Autodesk Inventor part; units mm, degrees
ref_plane "YZ Plane" through (0, 0, 0) normal (1, 0, 0) x (0, 1, 0)
ref_plane "XZ Plane" through (0, 0, 0) normal (0, 1, 0) x (-1, 0, 0)
ref_plane "XY Plane" through (0, 0, 0) normal (0, 0, 1) x (1, 0, 0)
sketch "스케치1" plane through (0, 0, 0) normal (0, 0, 1) x (1, 0, 0)
  arc A0 (0, 12.5) -> (-12.5, 0) centre (0, 0) ccw
  line L0 (0, 220.6094) -> (0, -371.145)
  line L1 (-77.086, -220) -> (-110, -35)
  line L2 (-110, -35) -> (-110, 15)
  spline S0 degree 2 poles (-110, 15) (-61.239, 69.4656) (0, 70) knots 0 0 0 1 1 1
  line L3 (-29.7943, 69.74) -> (29.7943, 70.26) construction
  line L4 (-12.5, 0) -> (-12.5, -190)
  line L5 (-12.5, -190) -> (-29.9689, -220)
  line L6 (-29.9689, -220) -> (-77.086, -220)
  arc A1 (12.5, 0) -> (0, 12.5) centre (0, 0) ccw
  line L7 (77.086, -220) -> (110, -35)
  line L8 (110, -35) -> (110, 15)
  spline S1 degree 2 poles (110, 15) (61.239, 69.4656) (0, 70) knots 0 0 0 1 1 1
  line L9 (29.7943, 69.74) -> (-29.7943, 70.26) construction
  line L10 (12.5, 0) -> (12.5, -190)
  line L11 (12.5, -190) -> (29.9689, -220)
  line L12 (29.9689, -220) -> (77.086, -220)
  point P0 (1.2114, -68.8044)
  point P1 (23.5091, 68.2027)
  point P2 (-23.4485, 67.5354)
  point P3 (-1.2114, -68.8044)
  point P4 (-23.5091, 68.2027)
  point P5 (23.4485, 67.5354)
  point P6 (0, 70)
  dimension "d0" = 25
  dimension "d3" = 110
  dimension "d4" = 50
  dimension "d5" = 190
  dimension "d8" = 70
  dimension "d25" = 290
extrude "Wheel Body Initial Extrusion" add sketch "스케치1" along normal mid plane 60
sketch "스케치4" plane through (-12.5, -190, 30) normal (1, 0, 0) x (0, 0, -1)
  line L0 (60, 190) -> (0, 190)
  line L1 (60, 190) -> (60, 0)
  line L2 (60, 0) -> (0, 0)
  line L3 (0, 0) -> (0, 190)
  line L4 (0, 190) -> (0, -93.6851)
  line L5 (23, 50) -> (10, 50)
  line L6 (10, 50) -> (10, -48.4584)
  line L7 (10, -10.6044) -> (23, -10.6044)
  line L8 (23, -10.6044) -> (23, -50.5115)
  line L9 (23, -50.5115) -> (0, -50.5115)
  line L10 (53, -93.6851) -> (53, 276.7845)
  line L11 (53, 190) -> (0, 190)
  line L12 (53, 259.8429) -> (0, 259.8429)
  line L13 (0, 259.8429) -> (0, 0)
  point P0 (30, 190)
  dimension "d18" = 13
  dimension "d19" = 140
  dimension "d20" = 7
sketch "스케치7" plane through (0, 0, 30) normal (0, 0, 1) x (1, 0, 0)
  line L0 (-103, -34.3822) -> (-71.2215, -213)
  line L1 (-71.2215, -213) -> (-34.8207, -213)
  line L2 (-29.9689, -220) -> (-77.086, -220)
  line L3 (-34.8207, -213) -> (-19.5, -189.0198)
  line L4 (-19.5, -189.0198) -> (-19.5, 0)
  line L5 (-103, -34.3822) -> (-103, 27.8234)
  line L6 (-103, 27.8234) -> (-55.0885, 51.7889) construction
  line L7 (-55.0885, 51.7889) -> (35.24, 53.8015) construction
  spline S0 degree 2 poles (-103, 27.8234) (-55.0885, 51.7889) (35.24, 53.8015) knots 1 1 1 2 2 2
  line L8 (12.5, -190) -> (12.5, 0)
  arc A0 (12.5, 0) -> (-12.5, 0) centre (0, 0) ccw
  line L9 (-110, 15) -> (-110, -35)
  line L10 (-110, -35) -> (-77.086, -220)
  line L11 (-12.5, -190) -> (-12.5, 0)
  arc A1 (0, 19.5) -> (-19.5, 0) centre (0, 0) ccw
  line L12 (138.0234, -13.4315) -> (72.0365, -213)
  line L13 (72.0365, -213) -> (34.8207, -213)
  line L14 (34.8207, -213) -> (19.5, -189.0198)
  line L15 (19.5, -189.0198) -> (19.5, 0)
  line L16 (138.0234, -13.4315) -> (173.48, 27.8234)
  line L17 (173.48, 27.8234) -> (125.5685, 51.7889) construction
  line L18 (125.5685, 51.7889) -> (35.24, 53.8015) construction
  spline S1 degree 2 poles (173.48, 27.8234) (125.5685, 51.7889) (35.24, 53.8015) knots 1 1 1 2 2 2
  arc A2 (19.5, 0) -> (0, 19.5) centre (0, 0) ccw
  line L19 (72.0365, 0) -> (72.0365, -130)
  line L20 (106.0933, -110) -> (19.5, -110)
  line L21 (92.8673, -150) -> (19.5, -150)
  point P0 (-103, -3.2794)
  dimension "d40" = 7
  dimension "d42" = 7
  dimension "d43" = 7
  dimension "d44" = 7
  dimension "d53" = 130
  dimension "d54" = 20
  dimension "d57" = 40
extrude "Extrusion Cut for Thickness" [suppressed]
sketch "스케치8" plane through (110, -35, 30) normal (1, 0, 0) x (0, 0, -1)
  line L0 (60, 50) -> (60, 0)
  line L1 (60, 50) -> (30, 50)
  line L2 (60, 20) -> (60, 50)
  circle A0 centre (30, 35) radius 8.5
  dimension "d84" = 17
extrude "돌출3" [suppressed]
extrude "돌출4" [suppressed]
mirror "미러1" [suppressed]
extrude "돌출5" add sketch "스케치7" against normal blind 23 contours L12 L21 L15 L20
mirror "미러2" about plane through (0, 0, 0) normal (1, 0, 0) of "돌출5"
sketch "스케치21" plane through (0, 0, -30) normal (0, 0, -1) x (-1, 0, 0)
  line L0 (-77.086, -220) -> (-110, -35)
  line L1 (-110, -35) -> (-85, -35)
  line L2 (-85, -35) -> (-37.5, -92.3904)
  line L3 (-37.5, -92.3904) -> (-12.5, -92.3904)
  line L4 (-12.5, 0) -> (-12.5, -190)
  line L5 (0, 75.7954) -> (0, -227.3908)
  line L6 (110, -35) -> (85, -35)
  line L7 (85, -35) -> (37.5, -92.3904)
  line L8 (37.5, -92.3904) -> (12.5, -92.3904)
  line L9 (-110, -35) -> (-77.086, -220)
  line L10 (-29.9689, -220) -> (-77.086, -220)
  line L11 (-12.5, -190) -> (-29.9689, -220)
  line L12 (-29.9689, -220) -> (-12.5, -190)
  line L13 (-12.5, -190) -> (-12.5, -92.3904)
  line L14 (12.5, -92.3904) -> (12.5, -190)
  line L15 (29.9689, -220) -> (12.5, -190)
  line L16 (12.5, -190) -> (29.9689, -220)
  line L17 (110, -35) -> (77.086, -220)
  line L18 (29.9689, -220) -> (77.086, -220)
  line L19 (77.086, -220) -> (110, -35)
  point P0 (0, 0)
  dimension "d80" = 25
  dimension "d81" = 25
extrude "돌출9" cut sketch "스케치21" against normal blind 60
sketch "스케치22" plane through (110, 15, 30) normal (1, 0, 0) x (0, 0, -1)
  line L0 (60, -15) -> (0, -15)
  circle A0 centre (38.7205, -15) radius 8.5
  point P0 (30, -15)
  dimension "d86" = 17
extrude "돌출10" cut sketch "스케치22" against normal blind 80
sketch "스케치23" plane through (85, -35, -30) normal (0, -1, 0) x (1, 0, 0)
  circle A0 centre (12.5, 45) radius 8.5
  line L0 (25, 0) -> (25, 60)
  line L1 (0, 60) -> (25, 60)
  point P0 (-85, 30)
  dimension "d89" = 12.5
  dimension "d90" = 17
  dimension "d91" = 15
extrude "돌출11" cut sketch "스케치23" against normal blind 40
sketch "스케치24" plane through (12.5, -92.3904, -30) normal (0, -1, 0) x (1, 0, 0)
  circle A0 centre (-37.5, 28) radius 8.5
  circle A1 centre (85, 45) radius 8.5
  line L0 (-50, 0) -> (-50, 60)
  point P0 (-12.5, 30)
  dimension "d94" = 17
  dimension "d95" = 17
  dimension "d98" = 12.5
extrude "돌출12" cut sketch "스케치24" against normal blind 60 contours A0
ref_plane "작업 평면6" through (0, 0, -30) normal (-1, 0, 0) x (0, 0, 1)
mirror "미러4" about plane through (0, 0, -30) normal (-1, 0, 0) of "돌출10", "돌출11", "돌출12"
sketch "스케치25" plane through (-106.0933, -110, 7) normal (-0.9494, -0.3139, 0) x (0, 0, 1)
  point P0 (-7, 71.1329)
sketch "스케치26" plane through (0, 0, -30) normal (-1, 0, 0) x (0, 0, 1)
  line L0 (94.4532, -100.7618) -> (-29.2969, -100.7618)
  line L1 (-29.2969, -100.7618) -> (-29.2969, -183.2619)
  line L2 (-29.2969, -183.2619) -> (94.4532, -183.2619)
  line L3 (94.4532, -183.2619) -> (94.4532, -100.7618)
  point P0 (30, 0)
extrude "돌출13" cut sketch "스케치26" along normal mid plane 574.75
sketch "스케치27" plane through (0, 0, 30) normal (0, 0, 1) x (1, 0, 0)
  line L0 (80, -28.4941) -> (80, 31.156)
  line L1 (89, -35) -> (89, 5)
  line L2 (37.5, -92.3904) -> (85, -35)
  line L3 (85, -35) -> (85, 52.6509)
  line L4 (33.5, -32.3904) -> (33.5, -92.3904)
  line L5 (85, -22.453) -> (42.2581, -74.0946)
  line L6 (110, -8.5) -> (30, -8.5)
  line L7 (80, 31.156) -> (61.3028, 45.0673) construction
  line L8 (61.3028, 45.0673) -> (26.6107, 51.872) construction
  spline S0 degree 2 poles (80, 31.156) (61.3028, 45.0673) (26.6107, 51.872) knots 1 1 1 2 2 2
  line L9 (42.2581, -74.0946) -> (42.2581, -8.5) construction
  line L10 (42.2581, -8.5) -> (26.6107, 51.872) construction
  spline S1 degree 2 poles (42.2581, -74.0946) (42.2581, -8.5) (26.6107, 51.872) knots 1 1 1 2 2 2
  point P0 (0, 0)
  dimension "d102" = 8
  dimension "d103" = 5
extrude "돌출14" cut sketch "스케치27" against normal blind 53 contours L5 S1 L6 L0 | L6 S1 S0 L0
mirror "미러5" about plane through (0, 0, -30) normal (-1, 0, 0) of "돌출14"
properties part number "5th Wheel Body"
Verification items for the finished model (mm, model axes). A direction names the side the tool comes from. Coordinates: 2 decimals unless noted, no trailing zeros. Loops run counter-clockwise (first coordinate to the right, second up) from the corner with the lowest first, then second, coordinate; pieces in that order, holes last. Notation, with made-up numbers: (71, -29.5) -> (85, -29.5) arc R28 cw to (85, -3.5) -> close; hole circle Ø6 at (24, 67). An arc over 180 degrees is marked (long way). Answer in a Markdown table with one row per item. Add a question column.
1. Depth check by flat-ended pin: P1, Ø13.5, axis at y = 0, z = -8.72, coming from the -X side; P2, Ø20, axis at x = 98.5, z = 0, coming from the -Y side; P3, Ø19.5, axis at y = 0, z = -8.72, coming from the -X side; P4, Ø1.5, axis at x = 75, z = 8, coming from the +Y side. Enter the tip coordinate at first touch or a pass-through.
2. Section check B-B, the plane z = 15. Give the number of separate pieces and of enclosed holes in the cut face, then the cut area to 3 significant figures.
3. Access from +Z, -Z, +X, -X, +Y, -Y to the whole of each face (thin tool, end or side, straight path). Record for faces 4 (the face through (-98, -35, 0)), 5 (the face through (-26.84, -62.81, -10.3)), 6 (the face through (98, -35, 0)), 7 (the face through (-80, 2, 4)).
4. Section check A-A, the plane y = -80.5. Enter the section's corners in (x, z).
5. Draft check along X on faces 1 (the face through (-61.583, -63.293, -0.42)), 2 (the face through (97, 5, 15)), 3 (the face through (95.21, 5.745, -2.456)). Enter one of: +X half, -X half, draft (parallel to the pull), parting line (faces both ways), or undercut.
6. Material ranges on probe 1 along Z at (x, y) = (-36, 0); probe 2 along X at (y, z) = (35, 5.5); probe 3 along X at (y, z) = (17.5, 15), recorded low to high. Write a range as [from, to].
Derived:
| question | item | result |
|---|---|---|
| 1 | P1 | stops at x = -30 |
| 1 | P2 | stops at y = -35 |
| 1 | P3 | stops at x = -110 |
| 1 | P4 | stops at y = 46.58 |
| 2 | separate pieces | 1 |
| 2 | enclosed holes | 2 |
| 2 | area | 14,200 mm² |
| 3 | face 4 | +Z, -Z, -X, -Y |
| 3 | face 5 | -Y |
| 3 | face 6 | +Z, -Z, +X, -Y |
| 3 | face 7 | +Z |
| 4 | outline | (-47.34, -30) -> (-12.5, -30) -> (-12.5, 30) -> (-47.34, 30) -> close; (12.5, -30) -> (47.34, -30) -> (47.34, 30) -> (12.5, 30) -> close; hole circle Ø17 at (-25, -2); hole circle Ø17 at (25, -2) |
| 5 | face 1 | -X half |
| 5 | face 2 | undercut |
| 5 | face 3 | draft |
| 6 | probe 1 | z = [-30, -17.22], [-0.22, 30] |
| 6 | probe 2 | x = [-89.56, -74.31], [-30.66, 30.66], [74.31, 89.56] |
| 6 | probe 3 | x = [-107.73, -80], [-34.17, 34.17], [80, 107.73] |
